Work out the finished part from the listing and answer in its coordinate system (mm). A direction names the side the tool comes from. Give positions to 0.01 mm unless a question says otherwise; leave off trailing zeros. Loops run counter-clockwise (first coordinate to the right, second up) from the corner with the lowest first, then second, coordinate; pieces in that order, holes last.
from build123d import *

# Parameters (mm, degrees)
F0_R     = 5
F1_DEPTH = 95


with BuildPart() as f1:
    # F0 (on Front) → F1 (new body, symmetric)
    with BuildSketch(Plane.XZ):
        Polygon((-275, 75), (-275, -275), (275, -275), (275, 275), (-75, 275), align=None)
        with Locations((-267.5, -267.5)):
            Circle(F0_R, mode=Mode.SUBTRACT)
        with Locations((267.5, -267.5)):
            Circle(F0_R, mode=Mode.SUBTRACT)
        with Locations((-267.5, 71.8933982822)):
            Circle(F0_R, mode=Mode.SUBTRACT)
        with Locations((-71.8933982822, 267.5)):
            Circle(F0_R, mode=Mode.SUBTRACT)
        Polygon((260, -260), (-260, -260), (-260, 68.7867965644), (-68.7867965644, 260), (-35, 260), (260, 260), (260, 130), (260, -35), align=None, mode=Mode.SUBTRACT)
        with Locations((267.5, 267.5)):
            Circle(F0_R, mode=Mode.SUBTRACT)
    extrude(amount=F1_DEPTH, both=True)


solid = f1.part
Item 1: Find section A-A, the plane x = 184. Write down the section's boundary in (y, z).
Item 2: For faces 1 (the face through (93, -1, 260)), 2 (the face through (-174, -1, 176)), determine the directions among +Z, -Z, +X, -X, +Y, -Y from which every point of the face is accessible in a straight line to the end or side of a thin tool.
Item 3: Consider line 1 (X direction, y = -4, z = -267.5); line 2 (X direction, y = 73, z = -104). Determine where each line is inside the solid, lowest interval first.
Item 4: Determine the mould class of faces 3 (the face through (4, -1, -260)), 4 (the face through (-275, -1, -98)), 5 (the face through (19, -95, -264)), 6 (the face through (-260, 1, -98)) for opening direction X: released by +X, released by -X, zero draft, split by the parting line, or undercut.
Item 5: Find section C-C, the plane y = -54.5. Write down the section's boundary in (x, z).
Item 6: Flat-ended cylindrical pins translate along their axes: pin 1 Ø8 at (x, z) = (267.5, 267.5) entering from +Y; pin 2 Ø12 at (x, y) = (-154, -53.5) entering from +Z; pin 3 Ø4 at (y, z) = (-61.5, 156.5) entering from -X; pin 4 Ø16 at (x, z) = (-267.5, 71.89) entering from -Y. Find the tip coordinate at first contact, or state that the pin passes through.
Item 7: Find section B-B, the plane z = 203. Write down the section's boundary in (x, y).
Ans:
1. outline: (-95, -275) - (95, -275) - (95, -260) - (-95, -260) - close; (-95, 260) - (95, 260) - (95, 275) - (-95, 275) - close
2. face 1: +Y, -Y
2. face 2: +Z, -X, +Y, -Y
3. line 1: x = -275 to -272.5, -262.5 to 262.5, 272.5 to 275
3. line 2: x = -275 to -260, 260 to 275
4. face 3: undercut
4. face 4: released by -X
4. face 5: zero draft
4. face 6: undercut
5. outline: (-275, -275) - (275, -275) - (275, 275) - (-75, 275) - (-275, 75) - close; hole circle Ø10 at (-267.5, -267.5); hole circle Ø10 at (-267.5, 71.89); hole (-260, -260) - (260, -260) - (260, 260) - (-68.79, 260) - (-260, 68.79) - close; hole circle Ø10 at (-71.89, 267.5); hole circle Ø10 at (267.5, -267.5); hole circle Ø10 at (267.5, 267.5)
6. pin 1: passes through
6. pin 2: stops at z = 202
6. pin 3: stops at x = -195.5
6. pin 4: stops at y = -95
7. outline: (-147, -95) - (-125.79, -95) - (-125.79, 95) - (-147, 95) - close; (260, -95) - (275, -95) - (275, 95) - (260, 95) - close
